Part print with two shaded views. Sizes in mm from the minimum x, y, z corner. A direction names the side the tool comes from. Coordinates: 2 decimals unless noted, no trailing zeros. Loops run counter-clockwise (first coordinate to the right, second up) from the corner with the lowest first, then second, coordinate; pieces in that order, holes last.
(1) Slice it at D-D (x = 22.5). Give the cut face in (y, z).
(2) Tool access for the marked faces 1, 2, 3, 4 and 5: list every direction of +Z, -Z, +X, -X, +Y, -Y with a clear straight run to the whole face (end or side of a thin tool).
(3) Wall check: L1, parallel to Z at x = 21.75, y = 2.55; L2, parallel to X at y = 4.35, z = 2.7. Give the ranges that are in metal, low to high.
(4) Flat gauge pins, fed straight in: P1, Ø1.6, axis at x = 24, y = 3, coming from the -Z side; P2, Ø0.5, axis at y = 4, z = 2.5, coming from the +X side; P3, Ø2.5, axis at x = 25, z = 2, coming from the -Y side; P4, Ø1, axis at x = 10.5, z = 2.5, coming from the -Y side (3 decimals). Where does each tip first touch, or does it go through?
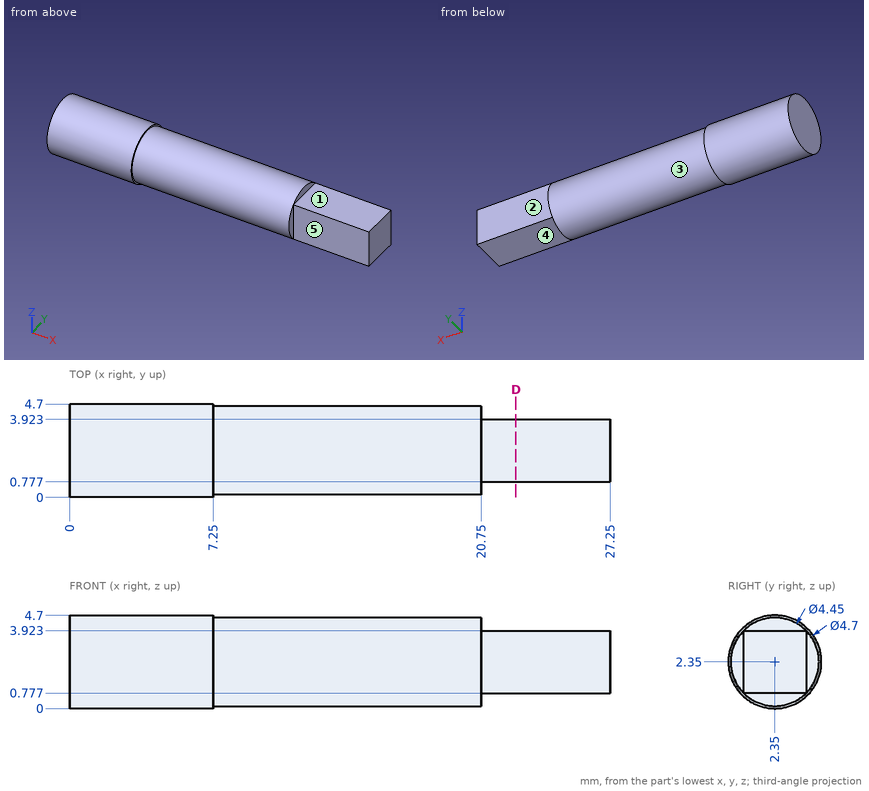
Response values:
1. outline: (0.78, 0.78) - (3.92, 0.78) - (3.92, 3.92) - (0.78, 3.92) - close
2. face 1: +Z, +X, +Y, -Y
2. face 2: +Z, -Z, +X, +Y
2. face 3: +X
2. face 4: -Z, +X, +Y, -Y
2. face 5: +Z, -Z, +X, -Y
3. L1: z = 0.78 to 3.92
3. L2: x = 0 to 20.75
4. P1: stops at z = 0.78
4. P2: stops at x = 27.25
4. P3: stops at y = 0.78
4. P4: stops at y = 0.125
